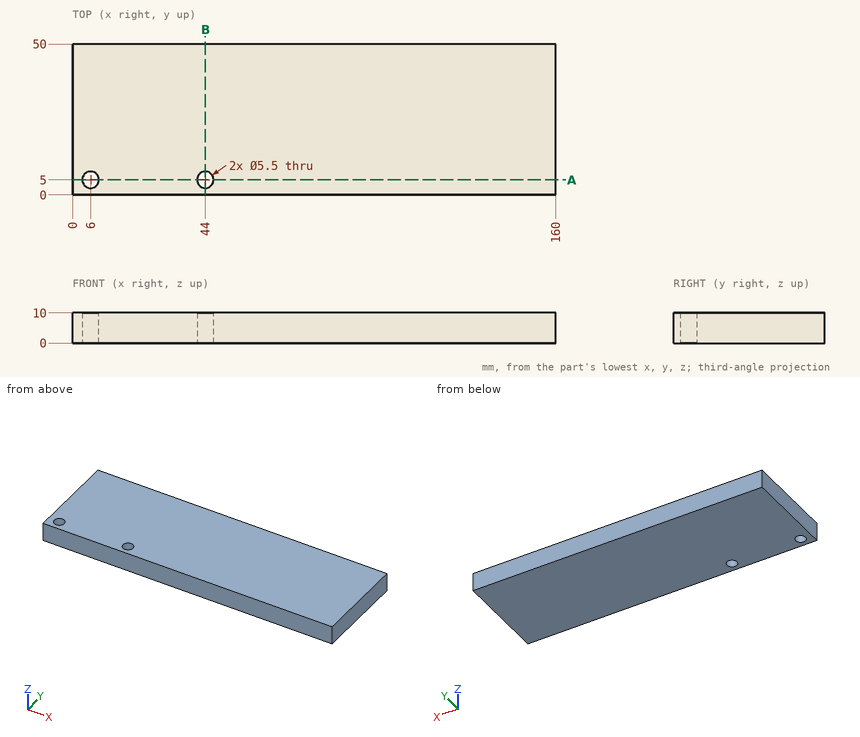
The figure shows three views and two pictorial views of one solid part (mm, origin at its lowest corner). Answer the questions. Coordinates: 2 decimals unless noted, no trailing zeros. Write each loop counter-clockwise with the first axis right and the second up, starting at its lowest first coordinate (ties: lowest second). Pieces come first, ordered by that corner, then holes. Notation, with made-up numbers: (-36, 70.25) -> (4, 70.25) arc R29 cw to (4, 98.25) -> close; hole circle Ø1 at (-12.5, 32.5). An arc over 180 degrees is marked (long way). Answer as a JSON object with one key per item and string values.
Q1. Consider line 1 (Y direction, x = 6, z = 4.25); line 2 (X direction, y = 6.5, z = 1.5). Determine where each line is inside the solid, lowest interval first. Write a range as [from, to].
The answers:
{"line 1": "y = [0, 2.25], [7.75, 50]", "line 2": "x = [0, 3.7], [8.3, 41.7], [46.3, 160]"}
Q2. The part is cut by section B-B on x = 44. Give the vertices of the cut face in (y, z), then the cut area to 3 significant figures.
The answers:
{"outline": "(0, 0) -> (2.25, 0) -> (2.25, 10) -> (0, 10) -> close; (7.75, 0) -> (50, 0) -> (50, 10) -> (7.75, 10) -> close", "area": "445 mm2"}
Q3. The part is cut by section A-A on y = 5. Give the vertices of the cut face in (x, z).
The answers:
{"outline": "(0, 0) -> (3.25, 0) -> (3.25, 10) -> (0, 10) -> close; (8.75, 0) -> (41.25, 0) -> (41.25, 10) -> (8.75, 10) -> close; (46.75, 0) -> (160, 0) -> (160, 10) -> (46.75, 10) -> close"}
